Verification items for the finished model (mm, model axes). A direction names the side the tool comes from. Coordinates: 2 decimals unless noted, no trailing zeros. Write each loop counter-clockwise with the first axis right and the second up, starting at its lowest first coordinate (ties: lowest second). Pieces come first, ordered by that corner, then holes. Notation, with made-up numbers: M 65.25,78.5 L 88.25,78.5 A7 cw 88.25,91.5 Z; hole C -39.5,-23 d9. An arc over 180 degrees is marked long. One line per item, written item: value.
```python
from build123d import *

# Parameters (mm, degrees)
SKETCH2_W               = 50.8
SKETCH2_H               = 19.05
BOSS_EXTRUDE1_DEPTH     = 4.445
CUT_EXTRUDE1_DEPTH      = 33.29387358
CUT_EXTRUDE1_DEPTH_BACK = 3.175
SKETCH4_W               = 33.02
SKETCH4_H               = 12.7
SKETCH6_W               = 22.86
SKETCH6_H               = 12.7
CUT_EXTRUDE2_DEPTH      = 29.546763827
FILLET2_R               = 9.525
SKETCH9_R               = 3.302
CUT_EXTRUDE4_DEPTH      = 29.546763827
SKETCH10_W              = 19.05
SKETCH10_H              = 19.05
BOSS_EXTRUDE2_DEPTH     = 3.175
FILLET1_R               = 2.54
SKETCH11_R              = 3.81
BOSS_EXTRUDE3_DEPTH     = 12.7
BOSS_EXTRUDE4_START     = 6.35
SKETCH12_R              = 3.81
BOSS_EXTRUDE4_DEPTH     = 6.35
SKETCH13_R              = 4.445
BOSS_EXTRUDE5_DEPTH     = 0.635
SKETCH14_R              = 5.08
BOSS_EXTRUDE6_DEPTH     = 5.08
BOSS_EXTRUDE7_DEPTH     = 5.08
CIRPATTERN1_COUNT       = 8
BOSS_EXTRUDE8_START     = 1.27
SKETCH16_R              = 4.445
BOSS_EXTRUDE8_DEPTH     = 1.27


# Some blends are built 0.0001 mm under size
with BuildPart() as part:
    # Sketch2 → Boss-Extrude1 (new, symmetric)
    with BuildSketch(Plane.XY):
        Rectangle(SKETCH2_W, SKETCH2_H)
    extrude(amount=BOSS_EXTRUDE1_DEPTH, both=True)

    # Sketch4 → Cut-Extrude1 (cut, two sides: drawn at the far end of the back side and taken through both)
    with BuildSketch(Plane(origin=(2.106978659, 4.870426214, 4.445), x_dir=(1, 0, 0), z_dir=(0, 0, 1)).offset(-CUT_EXTRUDE1_DEPTH_BACK)):
        with Locations((-8.456978659, -4.870426214)):
            Rectangle(SKETCH4_W, SKETCH4_H)
    extrude(amount=CUT_EXTRUDE1_DEPTH + CUT_EXTRUDE1_DEPTH_BACK, mode=Mode.SUBTRACT)

    # Sketch6 → Cut-Extrude2 (cut, through all)
    with BuildSketch(Plane(origin=(0, 0, -4.445), x_dir=(-1, 0, 0), z_dir=(0, 0, -1))):
        with Locations((6.35, 0)):
            Rectangle(SKETCH6_W, SKETCH6_H)
    extrude(amount=-CUT_EXTRUDE2_DEPTH, mode=Mode.SUBTRACT)

    # Fillet2
    fillet2_edges = [part.edges().sort_by_distance(p)[0] for p in [
        (25.4, -9.525, 0),
        (25.4, 9.525, 0),
    ]]
    fillet(fillet2_edges, radius=FILLET2_R - 0.0001)  # a hair under: the kernel refuses the full size

    # Sketch9 → Cut-Extrude4 (cut, through all)
    with BuildSketch(Plane.XY.offset(4.445)):
        with Locations((15.875, 0)):
            Circle(SKETCH9_R)
    extrude(amount=-CUT_EXTRUDE4_DEPTH, mode=Mode.SUBTRACT)

    # Sketch10 → Boss-Extrude2 (add)
    with BuildSketch(Plane(origin=(0, 9.525, 0), x_dir=(1, 0, 0), z_dir=(0, 1, 0))):
        with Locations((-7.62, 0)):
            Rectangle(SKETCH10_W, SKETCH10_H)
    extrude(amount=-BOSS_EXTRUDE2_DEPTH)

    # Fillet1
    # the kernel refuses this fillet: 2.54 mm, written as the material it adds along each edge
    with BuildSketch(Plane(origin=(-17.145, 9.525, -4.445), x_dir=(-1, 0, 0), z_dir=(0, -1, 0)), Plane(origin=(1.905, 6.35, -4.445), x_dir=(1, 0, 0), z_dir=(0, 1, 0))) as fillet1_piece_1:
        with BuildLine():
            CenterArc((FILLET1_R, FILLET1_R), FILLET1_R, 180, 90)
            Line((0, FILLET1_R), (0, 0))
            Line((0, 0), (FILLET1_R, 0))
        make_face()
    extrude(amount=3.175)
    with BuildSketch(Plane(origin=(1.905, 6.35, 4.445), x_dir=(1, 0, 0), z_dir=(0, 1, 0)), Plane(origin=(-17.145, 9.525, 4.445), x_dir=(-1, 0, 0), z_dir=(0, -1, 0))) as fillet1_piece_2:
        with BuildLine():
            CenterArc((FILLET1_R, -FILLET1_R), FILLET1_R, 90, 90)
            Line((0, -FILLET1_R), (0, 0))
            Line((0, 0), (FILLET1_R, 0))
        make_face()
    extrude(amount=3.175)
    # the kernel refuses this fillet: 2.54 mm, written as the material it takes off along each edge
    with BuildSketch(Plane(origin=(-25.4, -9.525, 10.795), x_dir=(1, 0, 0), z_dir=(0, 0, -1)), Plane(origin=(-25.4, 9.525, 10.795), x_dir=(0, -1, 0), z_dir=(0, 0, -1))) as fillet1_2_piece_1:
        with BuildLine():
            CenterArc((FILLET1_R, -FILLET1_R), FILLET1_R, 90, 90)
            Line((0, -FILLET1_R), (0, 0))
            Line((0, 0), (FILLET1_R, 0))
        make_face()
    extrude(amount=21.59, mode=Mode.SUBTRACT)
    with BuildSketch(Plane(origin=(-17.145, 15.875, -9.525), x_dir=(1, 0, 0), z_dir=(0, -1, 0)), Plane(origin=(1.905, 15.875, -9.525), x_dir=(0, 0, 1), z_dir=(0, -1, 0)), Plane(origin=(-17.145, 15.875, 9.525), x_dir=(0, 0, -1), z_dir=(0, -1, 0)), Plane(origin=(1.905, 15.875, 9.525), x_dir=(-1, 0, 0), z_dir=(0, -1, 0))) as fillet1_2_piece_2:
        with BuildLine():
            CenterArc((FILLET1_R, FILLET1_R), FILLET1_R, 180, 90)
            Line((0, FILLET1_R), (0, 0))
            Line((0, 0), (FILLET1_R, 0))
        make_face()
    extrude(amount=15.875, mode=Mode.SUBTRACT)

    # Sketch11 → Boss-Extrude3 (add)
    with BuildSketch(Plane(origin=(0, 9.525, 0), x_dir=(1, 0, 0), z_dir=(0, 1, 0))):
        with Locations(Location((-7.62, 0, 0), (0, 0, 90))):
            Circle(SKETCH11_R)
    extrude(amount=BOSS_EXTRUDE3_DEPTH)

    # Sketch12 → Boss-Extrude4 (add)
    with BuildSketch(Plane.XZ.offset(9.525).offset(BOSS_EXTRUDE4_START)):
        with Locations(Location((-7.62, 0, 0), (0, 0, 270))):
            Circle(SKETCH12_R)
    extrude(amount=-BOSS_EXTRUDE4_DEPTH)

    # Sketch13 → Boss-Extrude5 (add)
    with BuildSketch(Plane(origin=(0, 9.525, 0), x_dir=(1, 0, 0), z_dir=(0, 1, 0))):
        with Locations(Location((-7.62, 0, 0), (0, 0, 90))):
            Circle(SKETCH13_R)
    extrude(amount=BOSS_EXTRUDE5_DEPTH)

    # Sketch14 → Boss-Extrude6 (add)
    with BuildSketch(Plane(origin=(0, 10.16, 0), x_dir=(1, 0, 0), z_dir=(0, 1, 0))):
        with Locations(Location((-7.62, 0, 0), (0, 0, 270))):
            Circle(SKETCH14_R)
    extrude(amount=BOSS_EXTRUDE6_DEPTH)

    # Sketch15 → Boss-Extrude7 (add)
    with BuildSketch(Plane(origin=(0, 15.24, 0), x_dir=(1, 0, 0), z_dir=(0, 1, 0))):
        Polygon((-8.255, 7.62), (-6.985, 7.62), (-6.305199251, 4.906903198), (-8.934800749, 4.906903198), align=None)
    boss_extrude7 = extrude(amount=-BOSS_EXTRUDE7_DEPTH)

    # CirPattern1: Boss-Extrude7 ×8 about axis
    cirpattern1_axis = Axis((-7.62, 0, 0), (0, 1, 0))
    for i in range(1, CIRPATTERN1_COUNT):
        add(boss_extrude7.rotate(cirpattern1_axis, i * 360 / CIRPATTERN1_COUNT))

    # Sketch16 → Boss-Extrude8 (add)
    with BuildSketch(Plane.XZ.offset(9.525).offset(BOSS_EXTRUDE8_START)):
        with Locations(Location((-7.62, 0, 0), (0, 0, 270))):
            Circle(SKETCH16_R)
    extrude(amount=-BOSS_EXTRUDE8_DEPTH)


solid = part.part
```
Item 1: Draft check along X on faces 5 (the face through (-5.67, 12.66, -4.69)), 6 (the face through (-2.93, 12.66, 1.95)), 7 (the face through (-5, 15.24, -3)), 8 (the face through (-9.555, 12.664, -4.697)). Enter one of: released by +X, released by -X, zero draft, split by the parting line, or undercut.
The answers:
face 5: undercut
face 6: released by +X
face 7: zero draft
face 8: undercut
Item 2: Cross-section at C-C, the plane y = 5. Enter the section's corners in (x, z) (3 decimals), and give its area (3 significant figures).
The answers:
outline: M -25.4,-4.445 L -17.78,-4.445 L -17.78,1.27 L -22.86,1.27 L -22.86,4.445 L -25.4,4.445 Z; M 5.08,-4.445 L 23.982,-4.445 L 23.982,4.445 L 10.16,4.445 L 10.16,1.27 L 5.08,1.27 Z
area: 204 mm²
Item 3: Access from +Z, -Z, +X, -X, +Y, -Y to the whole of each face (thin tool, end or side, straight path). Record for faces 1 (the face through (-3.86, 12.74, 5.13)), 2 (the face through (-12.728, 12.736, -3.723)), 3 (the face through (-8, 13, 7.62)), 4 (the face through (-11.96, -10.17, 0.96)).
The answers:
face 1: +Z, +Y
face 2: -X, +Y
face 3: +Z, +X, -X, +Y
face 4: -Y
Item 4: Go/stop test with flat-tipped pins: P1, Ø1.5, axis at x = -1, y = 12, coming from the -Z side; P2, Ø1, axis at y = 11.5, z = -0.5, coming from the -X side; P3, Ø10, axis at x = -18.5, y = -7.5, coming from the +Z side (3 decimals). Record where each tip stops, or that it passes through.
The answers:
P1: stops at z = -1.07
P2: stops at x = -15.24
P3: stops at z = 4.445
Item 5: Cross-section at A-A, the plane z = 0. Give the number of separate pieces and of enclosed holes in the cut face, and give its area (3 significant figures).
The answers:
separate pieces: 1
enclosed holes: 2
area: 788 mm²
Item 6: Scan lines: line 1 (Y direction, x = -7, z = -3.5) (3 decimals); line 2 (Y direction, x = 3.5, z = -2.75) (3 decimals); line 3 (Y direction, x = 11, z = 1.5) (3 decimals). Record each from-to range of solid material in increasing order.
The answers:
line 1: y = -15.875 to -6.35, 6.35 to 22.225
line 2: y = -9.525 to -6.35, 6.35 to 9.525
line 3: y = -9.525 to 9.525
Item 7: Cross-section at B-B, the plane x = 3.5. Enter the section's corners in (y, z) (3 decimals).
The answers:
outline: M -9.525,-4.445 L -6.35,-4.445 L -6.35,4.445 L -9.525,4.445 Z; M 6.35,-4.627 L 9.525,-4.627 L 9.525,4.627 L 6.35,4.627 Z
Item 8: Cross-section at D-D, the plane y = -13. Enter the section's corners in (x, z), and give its area (3 significant figures).
The answers:
outline: C -7.62,0 d7.62
area: 45.6 mm²
